Verification items for the finished model (mm, model axes). Face numbers are marked on the shaded views. A direction names the side the tool comes from. Coordinates: 2 decimals unless noted, no trailing zeros. Order: outer loops, then holes, each group sorted by start corner. A loop starts at its lowest first (then second) coordinate and runs counter-clockwise, first axis right, second up. Notation, with made-up numbers: M -29.5,61 L 6.5,61 A16 ccw 6.5,76 Z; hole C 78,41 d6. An arc over 180 degrees is marked long. Write item = value, one per line.
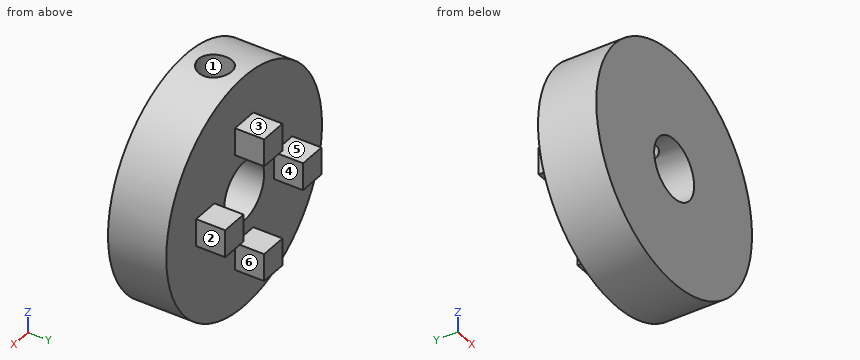
```python
from build123d import *

# Parameters (mm, degrees)
SKETCH1_R           = 20
SKETCH1_R_2         = 5.125
BOSS_EXTRUDE1_DEPTH = 10
SKETCH2_W           = 4.7
SKETCH2_H           = 4.7
BOSS_EXTRUDE2_DEPTH = 5
SKETCH3_R           = 2
CUT_EXTRUDE2_DEPTH  = 21
CUT_EXTRUDE3_START  = 10
SKETCH4_R           = 2.85
CUT_EXTRUDE3_DEPTH  = 11.000000127


with BuildPart() as part:
    # Sketch1 → Boss-Extrude1 (new body)
    with BuildSketch(Plane(origin=(0, 0, 0), x_dir=(1, 0, 0), z_dir=(0, 1, 0))):
        Circle(SKETCH1_R)
        Circle(SKETCH1_R_2, mode=Mode.SUBTRACT)
    extrude(amount=BOSS_EXTRUDE1_DEPTH)

    # Sketch2 → Boss-Extrude2 (add)
    with BuildSketch(Plane(origin=(0, 10, 0), x_dir=(1, 0, 0), z_dir=(0, 1, 0))):
        with Locations((10, 0)):
            Rectangle(SKETCH2_W, SKETCH2_H)
        with Locations((0, 10)):
            Rectangle(SKETCH2_W, SKETCH2_H)
        with Locations((0, -10)):
            Rectangle(SKETCH2_W, SKETCH2_H)
        with Locations((-10, 0)):
            Rectangle(SKETCH2_W, SKETCH2_H)
    extrude(amount=BOSS_EXTRUDE2_DEPTH)

    # Sketch3 → Cut-Extrude2 (cut, through all)
    with BuildSketch(Plane.XY):
        with Locations((0, 5)):
            Circle(SKETCH3_R)
    extrude(amount=CUT_EXTRUDE2_DEPTH, mode=Mode.SUBTRACT)

    # Sketch4 → Cut-Extrude3 (cut, through all)
    with BuildSketch(Plane.XY.offset(CUT_EXTRUDE3_START)):
        with Locations((0, 5)):
            Circle(SKETCH4_R)
    extrude(amount=CUT_EXTRUDE3_DEPTH, mode=Mode.SUBTRACT)


solid = part.part
```
Item 1: Scan lines: L1, parallel to Y at x = 0, z = 7.2; L2, parallel to X at y = 13.5, z = 0. Record each from-to range of solid material in increasing order. Write a range as from..to.
Report:
L1 = 0..3, 7..10
L2 = -12.35..-7.65, 7.65..12.35
Item 2: Gauge pin test, flat ends, axial feed: pin 1 (5 mm diameter, centred on x = -0.5, y = 13, fed in from +Z); pin 2 (3 mm diameter, centred on y = 2, z = 1, fed in from +X); pin 3 (2 mm diameter, centred on x = 5, y = 10, fed in from -Z); pin 4 (4.5 mm diameter, centred on x = 0, y = 5, fed in from +Z). Record the tip position at first contact, or that the pin passes through.
Report:
pin_1 = 12.35
pin_2 = 20
pin_3 = -19.6
pin_4 = 10
Item 3: Sectioned sample at D-D, the plane y = 9.25. Enter the section's corners in (x, z) (3 decimals).
Report:
outline = C 0,0 d40; hole C 0,0 d10.25
Item 4: Sectioned sample at A-A, the plane z = 0. Enter the section's corners in (x, y) (3 decimals), then the cut area to 4 significant figures.
Report:
outline = M -20,0 L -5.125,0 L -5.125,10 L -7.65,10 L -7.65,15 L -12.35,15 L -12.35,10 L -20,10 Z; M 5.125,0 L 20,0 L 20,10 L 12.35,10 L 12.35,15 L 7.65,15 L 7.65,10 L 5.125,10 Z
area = 344.5 mm^2
Item 5: Tool access check on the marked faces 1, 2 and 3. Record the directions out of +Z, -Z, +X, -X, +Y, -Y that give a thin tool (end or side, any length) a straight path to the whole face; none if there is none.
Report:
face_1 = +Z
face_2 = +Z, -Z, +X, +Y
face_3 = +Z, +X, -X, +Y
Item 6: Sectioned sample at C-C, the plane x = 0. Enter the section's corners in (y, z) (3 decimals), then the cut area to 3 significant figures.
Report:
outline = M 0,-20 L 10,-20 L 10,-12.35 L 15,-12.35 L 15,-7.65 L 10,-7.65 L 10,-5.125 L 0,-5.125 Z; M 0,5.125 L 3,5.125 L 3,10 L 2.15,10 L 2.15,20 L 0,20 Z; M 7,5.125 L 10,5.125 L 10,7.65 L 15,7.65 L 15,12.35 L 10,12.35 L 10,20 L 7.85,20 L 7.85,10 L 7,10 Z
area = 268 mm^2
Item 7: Sectioned sample at B-B, the plane y = 12.5. Enter the section's corners in (x, z), then the cut area to 3 significant figures.
Report:
outline = M -12.35,-2.35 L -7.65,-2.35 L -7.65,2.35 L -12.35,2.35 Z; M -2.35,-12.35 L 2.35,-12.35 L 2.35,-7.65 L -2.35,-7.65 Z; M -2.35,7.65 L 2.35,7.65 L 2.35,12.35 L -2.35,12.35 Z; M 7.65,-2.35 L 12.35,-2.35 L 12.35,2.35 L 7.65,2.35 Z
area = 88.4 mm^2
Item 8: Release check for a two-part mould opening along X. For the marked faces 4, 5 and 6 record: pulls with the +X half, pulls with the -X half, needs draft (parallel to the pull), parting line crosses it, or undercut.
Report:
face_4 = undercut
face_5 = needs draft
face_6 = pulls with the +X half
